Autodesk Inventor part; units mm, degrees
ref_plane "Work Plane1" through (-65, 43.5, 0) normal (0, 0, 1) x (0, -1, 0)
ref_plane "YZ Plane" through (0, 0, 0) normal (1, 0, 0) x (0, 1, 0)
ref_plane "XZ Plane" through (0, 0, 0) normal (0, 1, 0) x (-1, 0, 0)
sketch "Sketch1" plane through (0, 0, 0) normal (0, 0, 1) x (1, 0, 0)
  line L0 (0, 0) -> (-65, 0)
  line L1 (-65, 0) -> (-65, 43.5)
  line L2 (-65, 43.5) -> (0, 43.5)
  line L3 (0, 43.5) -> (0, 0)
  dimension "d0" = 43.5
  dimension "d1" = 65
extrude "Extrusion1" add sketch "Sketch1" along normal blind 60
sketch "Sketch2" plane through (0, 0, 0) normal (0, 0, -1) x (-1, 0, 0)
  line L0 (1.8, 41.7) -> (63.2, 41.7)
  line L1 (63.2, 41.7) -> (63.2, 1.8)
  line L2 (63.2, 1.8) -> (1.8, 1.8)
  line L3 (1.8, 1.8) -> (1.8, 41.7)
  line L4 (65, 43.5) -> (65, 0)
  line L5 (0, 43.5) -> (65, 43.5)
  line L6 (0, 0) -> (0, 43.5)
  line L7 (65, 0) -> (0, 0)
  point P0 (65, 21.75)
  dimension "d4" = 1.8
  dimension "d5" = 1.8
  dimension "d6" = 1.8
  dimension "d7" = 1.8
extrude "Extrusion2" cut sketch "Sketch2" against normal blind 58 contours L0 L1 L2 L3
fillet "Fillet1" radius 1 2 edges at (-65, 43.5, 30) (0, 43.5, 30)
sketch "Sketch5" plane through (0, 0, 60) normal (0, 0, 1) x (1, 0, 0)
  circle A0 centre (-32.5, 21.25) radius 8.5
  line L0 (-1, 43.5) -> (-64, 43.5)
  line L1 (-65, 42.5) -> (-65, 0)
  point P0 (0, 0)
  point P1 (-32.5, 43.5)
  point P2 (-65, 21.25)
  dimension "d41" = 17
extrude "Extrusion5" cut sketch "Sketch5" against normal blind 10
sketch "Sketch6" plane through (0, 0, 60) normal (0, 0, 1) x (1, 0, 0)
  line L0 (-47.5, 33.25) -> (-17.5, 33.25)
  line L1 (-17.5, 33.25) -> (-17.5, 9.25)
  line L2 (-17.5, 9.25) -> (-47.5, 9.25)
  line L3 (-47.5, 9.25) -> (-47.5, 33.25)
  line L4 (-1, 43.5) -> (-64, 43.5)
  line L5 (0, 0) -> (0, 42.5)
  circle A0 centre (-44.5, 32.25) radius 1.5
  circle A1 centre (-46.5, 29.75) radius 1.5
  line L6 (-32.5, 33.25) -> (-32.5, 9.25) construction
  line L7 (-47.5, 21.25) -> (-17.5, 21.25) construction
  line L8 (-17.5, 33.25) -> (-47.5, 33.25)
  line L9 (-17.5, 9.25) -> (-17.5, 33.25)
  circle A2 centre (-20.5, 32.25) radius 1.5
  circle A3 centre (-18.5, 29.75) radius 1.5
  circle A4 centre (-44.5, 10.25) radius 1.5
  circle A5 centre (-46.5, 12.75) radius 1.5
  circle A6 centre (-18.5, 12.75) radius 1.5
  circle A7 centre (-20.5, 10.25) radius 1.5
  point P0 (-32.5, 43.5)
  point P1 (0, 21.25)
  point P2 (-47.5, 9.25)
  point P3 (-17.5, 9.25)
  point P4 (-17.5, 9.25)
  point P5 (-47.5, 9.25)
  dimension "d44" = 30
  dimension "d45" = 24
  dimension "d46" = 3
  dimension "d47" = 3
  dimension "d49" = 1
  dimension "d50" = 1
  dimension "d53" = 8.5
  dimension "d54" = 12
extrude "Extrusion6" cut sketch "Sketch6" against normal up to surface (2 mm away) contours A1 L3 | L3 A1 | A5 L3 | L3 A5 | A3 L1 | L1 A3 | A6 L1 | L1 A6
sketch "Sketch7" plane through (0, 0, 60) normal (0, 0, 1) x (1, 0, 0)
  line L0 (-65, 42.5) -> (-65, 0)
  line L1 (-65, 42.5) -> (-70, 42.5)
  line L2 (-70, 42.5) -> (-70, 37.5)
  line L3 (-70, 37.5) -> (-65, 37.5)
  line L4 (-65, 37.5) -> (-65, 42.5)
  line L5 (0, 0) -> (0, 42.5)
  line L6 (0, 42.5) -> (5, 42.5)
  line L7 (5, 42.5) -> (5, 37.5)
  line L8 (5, 37.5) -> (0, 37.5)
  line L9 (0, 37.5) -> (0, 42.5)
  line L10 (-65, 0) -> (0, 0)
  line L11 (0, 0) -> (5, 0)
  line L12 (5, 0) -> (5, 5)
  line L13 (5, 5) -> (0, 5)
  line L14 (0, 5) -> (0, 0)
  line L15 (-65, 0) -> (-70, 0)
  line L16 (-70, 0) -> (-70, 5)
  line L17 (-70, 5) -> (-65, 5)
  line L18 (-65, 5) -> (-65, 0)
  circle A0 centre (-67.5, 40) radius 1.35
  circle A1 centre (-67.5, 2.5) radius 1.35
  circle A2 centre (2.5, 2.5) radius 1.35
  circle A3 centre (2.5, 40) radius 1.35
  dimension "d57" = 5
  dimension "d58" = 5
  dimension "d59" = 5
  dimension "d60" = 5
  dimension "d61" = 5
  dimension "d62" = 5
  dimension "d63" = 5
  dimension "d64" = 5
  dimension "d65" = 2.7
  dimension "d66" = 2.7
  dimension "d67" = 2.7
  dimension "d68" = 2.7
  dimension "d69" = 2.5
  dimension "d70" = 2.5
  dimension "d71" = 2.5
  dimension "d72" = 2.5
  dimension "d73" = 2.5
  dimension "d74" = 2.5
  dimension "d75" = 2.5
  dimension "d76" = 2.5
ref_plane "Work Plane1" through (-65, 43.5, 0) normal (0, 0, 1) x (0, -1, 0)
sketch "Sketch8" plane through (-65, 43.5, 0) normal (0, 0, 1) x (0, -1, 0)
  line L0 (6, 70) -> (6, 65)
  circle A0 centre (3.5, 67.5) radius 1.35
  line L1 (1, 70) -> (6, 70)
  line L2 (1, 65) -> (1, 70)
  line L3 (43.5, 65) -> (43.5, 70)
  circle A1 centre (41, 67.5) radius 1.35
  line L4 (43.5, 70) -> (38.5, 70)
  line L5 (38.5, 70) -> (38.5, 65)
  line L6 (43.5, 0) -> (43.5, -5)
  circle A2 centre (41, -2.5) radius 1.35
  line L7 (43.5, -5) -> (38.5, -5)
  line L8 (38.5, -5) -> (38.5, 0)
  line L9 (6, -5) -> (6, 0)
  circle A3 centre (3.5, -2.5) radius 1.35
  line L10 (1, -5) -> (6, -5)
  line L11 (1, 0) -> (1, -5)
  circle A4 centre (3.5, 67.5) radius 1.35
  circle A5 centre (41, 67.5) radius 1.35
  circle A6 centre (41, -2.5) radius 1.35
  circle A7 centre (3.5, -2.5) radius 1.35
  line L12 (1, 0) -> (43.5, 0)
  line L13 (1, 0) -> (6, 0)
  line L14 (6, 0) -> (6, -5)
  line L15 (6, -5) -> (1, -5)
  line L16 (1, -5) -> (1, 0)
  line L17 (38.5, 0) -> (43.5, 0)
  line L18 (43.5, 0) -> (43.5, -5)
  line L19 (43.5, -5) -> (38.5, -5)
  line L20 (38.5, -5) -> (38.5, 0)
  line L21 (38.5, 65) -> (43.5, 65)
  line L22 (43.5, 65) -> (43.5, 70)
  line L23 (43.5, 70) -> (38.5, 70)
  line L24 (38.5, 70) -> (38.5, 65)
  line L25 (43.5, 65) -> (1, 65)
  line L26 (1, 65) -> (6, 65)
  line L27 (6, 65) -> (6, 70)
  line L28 (6, 70) -> (1, 70)
  line L29 (1, 70) -> (1, 65)
extrude "Extrusion7" add sketch "Sketch8" along normal blind 5
full round fillet "Full Round Fillet5" first side at (-66.6667, 42.5, 1.6667) centre faces at (-70, 40.8333, 1.6667) second side at (-68.3333, 37.5, 1.6667)
full round fillet "Full Round Fillet6" first side at (-43.3333, 0, 23.3333) centre faces at (-70, 3.3333, 1.6667) second side at (-66.6667, 5, 1.6667)
full round fillet "Full Round Fillet7" first side at (1.6667, 42.5, 3.3333) centre faces at (5, 39.1667, 1.6667) second side at (1.6667, 37.5, 1.6667)
full round fillet "Full Round Fillet8" first side at (-43.3333, 0, 23.3333) centre faces at (5, 1.6667, 1.6667) second side at (3.3333, 5, 1.6667)
properties part number "CAMCOVER"
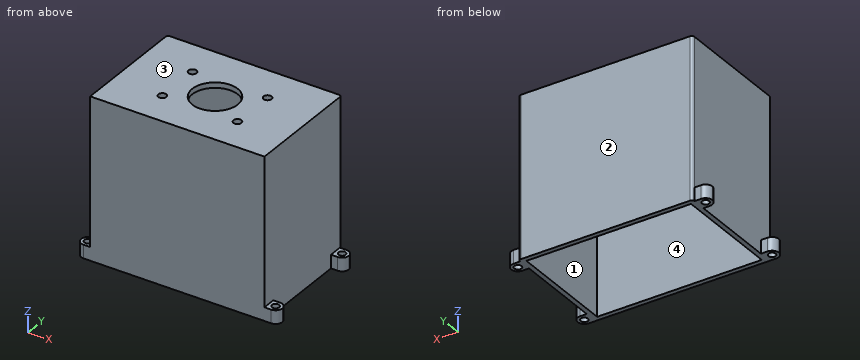
Can you work these out from the model? Positions are in its coordinate system, mm. Face numbers are marked on the shaded views. A direction names the side the tool comes from. Round coordinates to 2 decimals unless told otherwise and drop trailing zeros. Loops run counter-clockwise (first coordinate to the right, second up) from the corner with the lowest first, then second, coordinate; pieces in that order, holes last. Notation, with made-up numbers: (10.5, 40) -> (57.5, 40) arc R4 cw to (57.5, 45) -> close; hole circle Ø5 at (74, -38). An arc over 180 degrees is marked (long way). Answer in a Markdown table with one row per item.
Item 1: We'd pull the mould along X, two halves only. Please class the marked faces 1 and 2: released by +X, released by -X, zero draft, split by the parting line, or undercut.
Answer block:
| item | result |
|---|---|
| face 1 | undercut |
| face 2 | zero draft |
Item 2: Suppose I cut it at D-D, the plane x = -46.5. List the corners of the cut face in (y, z) for me, plus the area to 3 significant figures.
Answer block:
| item | result |
|---|---|
| outline | (0, 0) -> (1.8, 0) -> (1.8, 58) -> (11.25, 58) -> (11.25, 60) -> (0, 60) -> close; (14.25, 58) -> (28.25, 58) -> (28.25, 60) -> (14.25, 60) -> close; (31.25, 58) -> (41.7, 58) -> (41.7, 0) -> (43.5, 0) -> (43.5, 60) -> (31.25, 60) -> close |
| area | 284 mm² |
Item 3: Suppose I cut it at A-A, the plane x = -32.5. List the corners of the cut face in (y, z) for me, plus the area to 3 significant figures.
Answer block:
| item | result |
|---|---|
| outline | (0, 0) -> (1.8, 0) -> (1.8, 58) -> (12.75, 58) -> (12.75, 60) -> (0, 60) -> close; (29.75, 58) -> (41.7, 58) -> (41.7, 0) -> (43.5, 0) -> (43.5, 60) -> (29.75, 60) -> close |
| area | 262 mm² |
Item 4: Suppose I cut it at C-C, the plane y = 19. List the corners of the cut face in (x, z) for me, plus the area to 3 significant figures.
Answer block:
| item | result |
|---|---|
| outline | (-65, 0) -> (-63.2, 0) -> (-63.2, 58) -> (-40.7, 58) -> (-40.7, 60) -> (-65, 60) -> close; (-24.3, 58) -> (-1.8, 58) -> (-1.8, 0) -> (0, 0) -> (0, 60) -> (-24.3, 60) -> close |
| area | 306 mm² |
Item 5: If I drill on probe 1 along Y at (x, z) = (-18.5, 59.55); probe 2 along Y at (x, z) = (-67.5, 3.45); probe 3 along Y at (x, z) = (-32.5, 59.1), over which ranges is the centre line in solid material (lowest first)?
Answer block:
| item | result |
|---|---|
| probe 1 | 0 to 11.25, 14.25 to 28.25, 31.25 to 43.5 |
| probe 2 | 0 to 1.15, 3.85 to 5, 37.5 to 38.65, 41.35 to 42.5 |
| probe 3 | 0 to 12.75, 29.75 to 43.5 |
Item 6: On a 3-axis mill with a long thin cutter (end or side, diameter ignored), from which of +Z, -Z, +X, -X, +Y, -Y can I reach the whole of each face in a straight line? I mean the marked faces 3 and 4. Say none if no direction works.
Answer block:
| item | result |
|---|---|
| face 3 | +Z, +X, -X, +Y, -Y |
| face 4 | -Z |
Item 7: Suppose I cut it at B-B, the plane z = 14.5. List the corners of the cut face in (x, y) for me.
Answer block:
| item | result |
|---|---|
| outline | (-65, 0) -> (0, 0) -> (0, 42.5) arc R1 ccw to (-1, 43.5) -> (-64, 43.5) arc R1 ccw to (-65, 42.5) -> close; hole (-63.2, 1.8) -> (-1.8, 1.8) -> (-1.8, 41.7) -> (-63.2, 41.7) -> close |
Item 8: Will these pins go through, and if not, where does the flat tip stop? P1, Ø8, axis at y = 26, z = 25, coming from the -X side; P2, Ø1, axis at x = -50.5, y = 22.5, coming from the -Z side; P3, Ø1.3, axis at x = -66.5, z = 2.5, coming from the +Y side; P4, Ø1.8, axis at x = -18.5, y = 12.75, coming from the +Z side.
Answer block:
| item | result |
|---|---|
| P1 | x = -65 |
| P2 | z = 58 |
| P3 | y = 42.5 |
| P4 | through |
